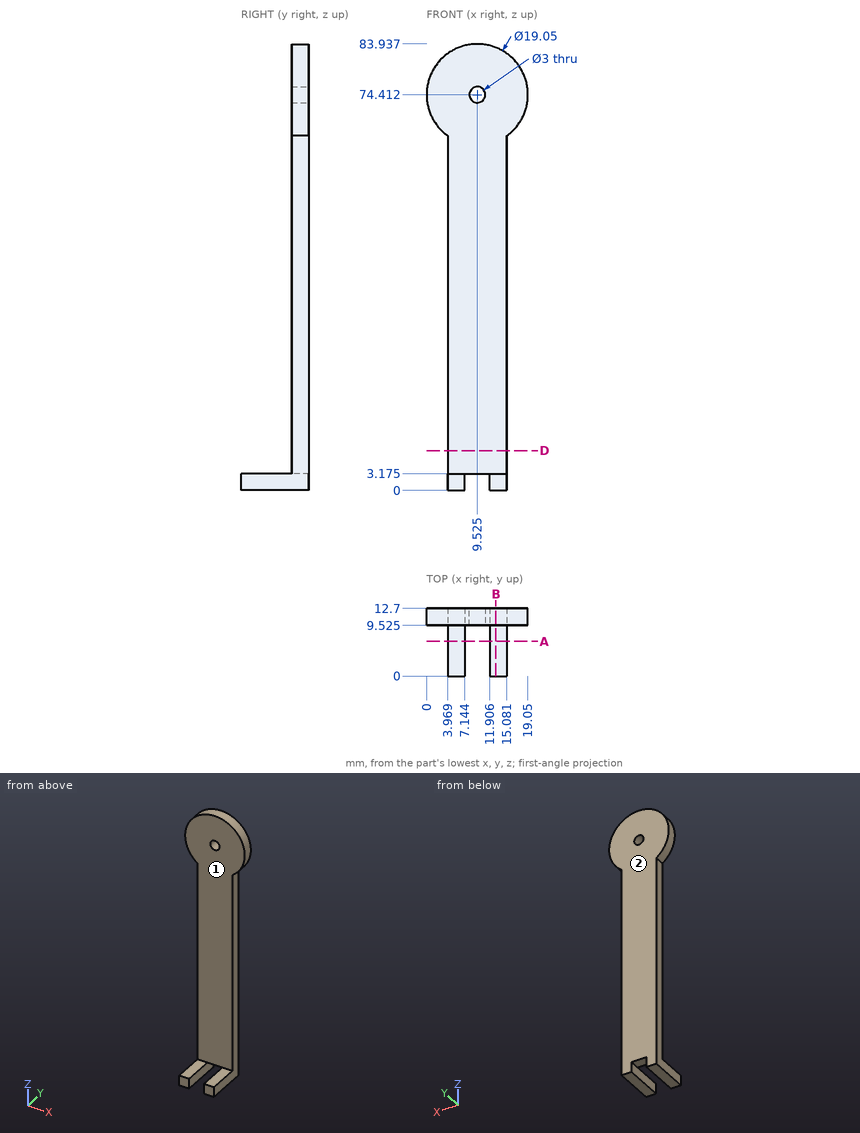
Geometry: see drawing. Coordinates: mm, zero at the bounding-box minimum. A direction names the side the tool comes from. Round coordinates to 2 decimals unless told otherwise and drop trailing zeros. Order: outer loops, then holes, each group sorted by start corner. A loop starts at its lowest first (then second) coordinate and runs counter-clockwise, first axis right, second up. Notation, with made-up numbers: (71, 89) - (85, 89) arc R33 cw to (85, 120) - close; hole circle Ø6 at (86.25, 5). An arc over 180 degrees is marked (long way). Use a Markdown table: item, result. Add a question column.
1. First-contact query: pin 1 (1.5 mm diameter, centred on y = 10.5, z = 10, fed in from +X); pin 2 (3.5 mm diameter, centred on x = 9.52, z = 74.41, fed in from -Y) (1 decimal); pin 3 (1 mm diameter, centred on x = 7.5, y = 8.5, fed in from +Z) (1 decimal). Flat tips, straight axial feed; report the tip coordinate or a pass-through.
2. Set-up query: the marked faces 1 and 2. Return all of +Z, -Z, +X, -X, +Y, -Y with unobstructed straight access to the full face (end or side cutting, diameter ignored); none if empty.
3. Line query: probe 1 along Y at (x, z) = (15.75, 71) (1 decimal); probe 2 along Z at (x, y) = (13.25, 9) (1 decimal); probe 3 along Z at (x, y) = (10, 11.25) (1 decimal). Output: solid intervals per line, ascending.
4. Section query B-B (x = 13). Return the cut outline in (y, z) (1 decimal).
5. Section query A-A (y = 6.5). Return the cut outline in (x, z) (1 decimal).
6. Section query D-D (z = 7.5). Return the cut outline in (x, y) (1 decimal).
Derived:
| question | item | result |
|---|---|---|
| 1 | pin 1 | x = 15.08 |
| 1 | pin 2 | y = 9.5 |
| 1 | pin 3 | z = 3.2 |
| 2 | face 1 | +Z, +X, -X, -Y |
| 2 | face 2 | +Z, -Z, +X, -X, +Y |
| 3 | probe 1 | 9.5 to 12.7 |
| 3 | probe 2 | 0 to 3.2 |
| 3 | probe 3 | 3.2 to 73, 75.8 to 83.9 |
| 4 | outline | (0, 0) - (12.7, 0) - (12.7, 83.3) - (9.5, 83.3) - (9.5, 3.2) - (0, 3.2) - close |
| 5 | outline | (4, 0) - (7.1, 0) - (7.1, 3.2) - (4, 3.2) - close; (11.9, 0) - (15.1, 0) - (15.1, 3.2) - (11.9, 3.2) - close |
| 6 | outline | (4, 9.5) - (15.1, 9.5) - (15.1, 12.7) - (4, 12.7) - close |
